The listing builds one solid part. Answer for the finished solid, in the listing's coordinates (mm). A direction names the side the tool comes from. Give positions to 0.01 mm unless a question says otherwise; leave off trailing zeros. Loops run counter-clockwise (first coordinate to the right, second up) from the corner with the lowest first, then second, coordinate; pieces in that order, holes last. Notation, with made-up numbers: M 23.5,23.5 L 53.5,23.5 A30 ccw 53.5,47.5 Z; hole C -38.5,67.25 d9. An arc over 180 degrees is marked long. One line per item, written item: value. Start each with the question number.
Q1. Flat-ended cylindrical pins translate along their axes: pin 1 (4 mm diameter, centred on y = -3.5, z = -16, fed in from +X); pin 2 (3 mm diameter, centred on y = 0, z = -30.44, fed in from -X); pin 3 (1.2 mm diameter, centred on y = 0, z = -2.5, fed in from +X). Find the tip coordinate at first contact, or state that the pin passes through.
Q2. For faces 4 (the flat face through (12.5, 0, -2)), 5 (the flat face through (7, -6.25, -17)), 6 (the flat face through (8.99, -3, -17)), determine the directions among +Z, -Z, +X, -X, +Y, -Y from which every point of the face is accessible in a straight line to the end or side of a thin tool.
Q3. A cutting plane is placed at C-C, the plane y = 2.25. Determine the outline of the cut face in (x, z).
Q4. The mould has two halves that part along Z. Classify faces 1 (the flat face through (12.5, 0, -30)), 2 (the flat face through (0, -3, -16)), 3 (the flat face through (13, 0, 0)): +Z half, -Z half, draft (parallel to the pull), parting line (faces both ways), or undercut.
Q5. Consider L1, parallel to Y at x = 20, z = -30.44; L2, parallel to Z at x = 18.5, y = 1.5; L3, parallel to Y at x = 3, z = -16.47. Determine where each line is inside the solid, lowest interval first.
Q6. A cutting plane is placed at A-A, the plane x = 16.25. Determine the outline of the cut face in (y, z).
Q7. A cutting plane is placed at D-D, the plane y = -5.25. Determine the outline of the cut face in (x, z).
Q8. A cutting plane is placed at B-B, the plane z = -16.47. Determine the outline of the cut face in (x, y), and give its area (3 significant figures).
from build123d import *

# Parameters (mm, degrees)
Y_KSEKLIK_EKSTR_ZYON1_DEPTH = 6.25
IZIM2_R                     = 1.25
KES_EKSTR_ZYON1_DEPTH       = 12.5
IZIM4_R                     = 3
KES_EKSTR_ZYON2_DEPTH       = 10


with BuildPart() as part:
    # Çizim1 → Yükseklik-Ekstrüzyon1 (new, symmetric)
    with BuildSketch(Plane(origin=(0, 0, 0), x_dir=(1, 0, 0), z_dir=(0, 1, 0))):
        Polygon((0, 0), (0, 32.94), (25, 32.94), (25, 27.94), (8.99, 27.94), (8.99, 5), (25, 5), (25, 0), align=None)
    extrude(amount=Y_KSEKLIK_EKSTR_ZYON1_DEPTH, both=True)

    # Çizim2 → Kes-Ekstrüzyon1 (cut)
    with BuildSketch(Plane(origin=(25, 0, 0), x_dir=(0, 0, -1), z_dir=(1, 0, 0))):
        with Locations((2.5, 0)):
            Circle(IZIM2_R)
    kes_ekstr_zyon1 = extrude(amount=-KES_EKSTR_ZYON1_DEPTH, mode=Mode.SUBTRACT)

    # Aynalama1: Kes-Ekstrüzyon1 across plane
    add(kes_ekstr_zyon1.mirror(Plane.XY.offset(-16.47)), mode=Mode.SUBTRACT)

    # Çizim4 → Kes-Ekstrüzyon2 (cut)
    with BuildSketch(Plane.ZY):
        with Locations((-16.47, 1.25)):
            Circle(IZIM4_R)
    extrude(amount=-KES_EKSTR_ZYON2_DEPTH, mode=Mode.SUBTRACT)


solid = part.part
Answer block:
1. pin 1: x = 8.99
1. pin 2: x = 0
1. pin 3: x = 12.5
2. face 4: +X
2. face 5: +Z, -Z, +X, -X, -Y
2. face 6: +X, +Y, -Y
3. outline: M 0,-32.94 L 25,-32.94 L 25,-27.94 L 8.99,-27.94 L 8.99,-19.3 L 0,-19.3 Z; M 0,-13.64 L 8.99,-13.64 L 8.99,-5 L 25,-5 L 25,0 L 0,0 Z
4. face 1: undercut
4. face 2: draft
4. face 3: +Z half
5. L1: -6.25 to -1.25, 1.25 to 6.25
5. L2: -32.94 to -27.94, -5 to 0
5. L3: -6.25 to -1.75, 4.25 to 6.25
6. outline: M -6.25,-32.94 L 6.25,-32.94 L 6.25,-27.94 L -6.25,-27.94 Z; M -6.25,-5 L 6.25,-5 L 6.25,0 L -6.25,0 Z; hole C 0,-30.44 d2.5; hole C 0,-2.5 d2.5
7. outline: M 0,-32.94 L 25,-32.94 L 25,-27.94 L 8.99,-27.94 L 8.99,-5 L 25,-5 L 25,0 L 0,0 Z
8. outline: M 0,-6.25 L 8.99,-6.25 L 8.99,-1.75 L 0,-1.75 Z; M 0,4.25 L 8.99,4.25 L 8.99,6.25 L 0,6.25 Z
8. area: 58.4 mm^2
